from build123d import *

# Parameters (mm, degrees)
F0_W      = 39
F0_H      = 15
F1_DEPTH  = 4
F2_R      = 7.5
F3_DEPTH  = 3.9
F4_R      = 4
F5_DEPTH  = 4.2
F6_R      = 1.6
F7_DEPTH  = 25
F8_R      = 1.45
F9_DEPTH  = 25
F10_R     = 7.5
F10_R_2   = 5.5
F11_DEPTH = 0.2


# Not quite as in the source:
# - a feature names something its author has since deleted; it is built from what else it names


with BuildPart() as f1:
    # F0 (on Top) → F1 (new body)
    with BuildSketch(Plane.XY):
        with Locations((19.5, 7.5)):
            Rectangle(F0_W, F0_H)
    extrude(amount=F1_DEPTH)

    # F2 (on face) → F3 (join)
    with BuildSketch(Plane.XY.offset(4)):
        with Locations((19.5, 7.5)):
            Circle(F2_R)
    extrude(amount=F3_DEPTH)

    # F4 (on face) → F5 (cut)
    with BuildSketch(Plane.XY.offset(7.9)):
        with Locations((19.5, 7.5)):
            Circle(F4_R)
    extrude(amount=-F5_DEPTH, mode=Mode.SUBTRACT)

    # F6 (on face) → F7 (cut)
    with BuildSketch(Plane.XY.offset(4)):
        with Locations((35.5, 7.5)):
            Circle(F6_R)
        with Locations((3.5, 7.5)):
            Circle(F6_R)
    extrude(amount=-F7_DEPTH, mode=Mode.SUBTRACT)

    # F8 (on face) → F9 (cut)
    with BuildSketch(Plane.XY.offset(3.7)):
        with Locations((19.5, 7.5)):
            Circle(F8_R)
    extrude(amount=-F9_DEPTH, mode=Mode.SUBTRACT)

    # F10 (on face) → F11 (cut)
    with BuildSketch(Plane.XY.offset(7.9)):
        with Locations((19.5, 7.5)):
            Circle(F10_R)
        with Locations((19.5, 7.5)):
            Circle(F10_R_2, mode=Mode.SUBTRACT)
    extrude(amount=-F11_DEPTH, mode=Mode.SUBTRACT)


solid = f1.part
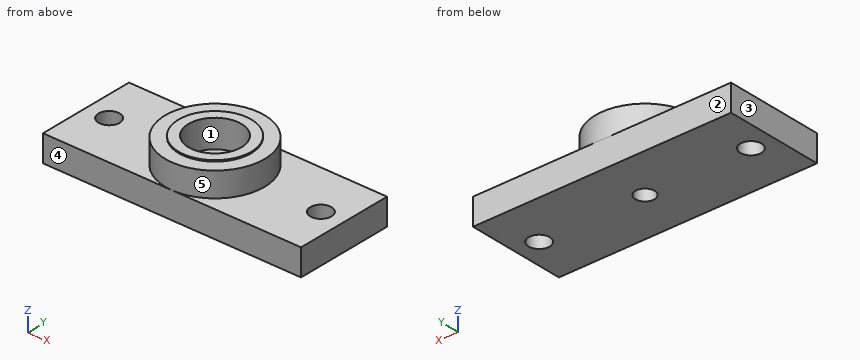
Input: part model. Units: mm. Frame: model coordinates. Face numbers are marked on the shaded views. A direction names the side the tool comes from. Coordinates: 2 decimals unless noted, no trailing zeros. Loops run counter-clockwise (first coordinate to the right, second up) from the corner with the lowest first, then second, coordinate; pieces in that order, holes last.
(1) Pull-direction query (X, two-part tool) for the marked faces 1, 2 and 3; classes: released by +X, released by -X, zero draft, split by the parting line, or undercut.
(2) Section D-D on x = 26.5. Return the cut outline in (y, z), then the cut area to 3 significant figures.
(3) Section A-A on x = 3.5. Return the cut outline in (y, z).
(4) Section B-B on y = 7.5. Return the cut outline in (x, z).
(5) Section C-C on z = 7. Return the cut outline in (x, y), then the cut area to 3 significant figures.
(6) Set-up query: the marked faces 4 and 5. Return all of +Z, -Z, +X, -X, +Y, -Y with unobstructed straight access to the full face (end or side cutting, diameter ignored); none if empty.
(7) First-contact query: pin 1 Ø1 at (y, z) = (4, 5) entering from +X; pin 2 Ø2.5 at (x, y) = (17.5, 6.5) entering from +Z; pin 3 Ø6.5 at (x, y) = (19.5, 7.5) entering from -Z; pin 4 Ø2 at (x, y) = (33.5, 12.5) entering from +Z. Flat tips, straight axial feed; report the tip coordinate or a pass-through.
(8) Material intervals for probe 1 along Y at (x, z) = (3.5, 1.5); probe 2 along Y at (x, z) = (19.5, 4.9); probe 3 along Z at (x, y) = (19.5, 4), sorted ascending.
Data:
1. face 1: undercut
1. face 2: zero draft
1. face 3: released by -X
2. outline: (0, 0) - (15, 0) - (15, 4) - (10.19, 4) - (10.19, 7.7) - (4.81, 7.7) - (4.81, 4) - (0, 4) - close
2. area: 79.9 mm2
3. outline: (0, 0) - (5.9, 0) - (5.9, 4) - (0, 4) - close; (9.1, 0) - (15, 0) - (15, 4) - (9.1, 4) - close
4. outline: (0, 0) - (1.9, 0) - (1.9, 4) - (0, 4) - close; (5.1, 0) - (18.05, 0) - (18.05, 3.7) - (15.5, 3.7) - (15.5, 7.9) - (14, 7.9) - (14, 7.7) - (12, 7.7) - (12, 4) - (5.1, 4) - close; (20.95, 0) - (33.9, 0) - (33.9, 4) - (27, 4) - (27, 7.7) - (25, 7.7) - (25, 7.9) - (23.5, 7.9) - (23.5, 3.7) - (20.95, 3.7) - close; (37.1, 0) - (39, 0) - (39, 4) - (37.1, 4) - close
5. outline: circle Ø15 at (19.5, 7.5); hole circle Ø8 at (19.5, 7.5)
5. area: 126 mm2
6. face 4: +Z, -Z, +X, -X, -Y
6. face 5: +Z
7. pin 1: stops at x = 26.37
7. pin 2: stops at z = 3.7
7. pin 3: stops at z = 0
7. pin 4: stops at z = 4
8. probe 1: y = 0 to 5.9, 9.1 to 15
8. probe 2: y = 0 to 3.5, 11.5 to 15
8. probe 3: z = 0 to 3.7
